from build123d import *

# Parameters (mm, degrees)
SKETCH1_R           = 50
SKETCH1_R_2         = 2.5
BOSS_EXTRUDE1_DEPTH = 3
SKETCH2_R           = 2
CUT_EXTRUDE1_DEPTH  = 4


with BuildPart() as part:
    # Sketch1 → Boss-Extrude1 (new body)
    with BuildSketch(Plane.XY):
        Circle(SKETCH1_R)
        Circle(SKETCH1_R_2, mode=Mode.SUBTRACT)
        with BuildLine():
            ThreePointArc((42, 0), (0, 42), (-42, 0))
            ThreePointArc((-42, 0), (-40, -2), (-38, 0))
            ThreePointArc((-38, 0), (0, 38), (38, 0))
            ThreePointArc((38, 0), (40, -2), (42, 0))
        make_face(mode=Mode.SUBTRACT)
    extrude(amount=BOSS_EXTRUDE1_DEPTH)

    # Sketch2 → Cut-Extrude1 (cut, through all)
    with BuildSketch(Plane.XY.offset(3)):
        with Locations((-15, 15)):
            Circle(SKETCH2_R)
        with Locations((15, 15)):
            Circle(SKETCH2_R)
        with Locations((15, -15)):
            Circle(SKETCH2_R)
        with Locations((-15, -15)):
            Circle(SKETCH2_R)
    extrude(amount=-CUT_EXTRUDE1_DEPTH, mode=Mode.SUBTRACT)


solid = part.part
Model file for the job. Use its own axes, mm. A direction names the side the tool comes from. Coordinates: 2 decimals unless noted, no trailing zeros. Loops run counter-clockwise (first coordinate to the right, second up) from the corner with the lowest first, then second, coordinate; pieces in that order, holes last. Notation, with made-up numbers: (35, 45.25) -> (93, 45.25) arc R23 cw to (93, 64.25) -> close; hole circle Ø7 at (32, 83). An arc over 180 degrees is marked (long way). Use one line per item in the form item = value. Start each with the question number.
(1) Flat gauge pins, fed straight in: pin 1 (6 mm diameter, centred on x = -25, y = 5, fed in from -Z); pin 2 (1 mm diameter, centred on y = -38.5, z = 2.5, fed in from +X). Where does each tip first touch, or does it go through?
(2) Probe probe 1 along Y at (x, z) = (15, 2.15); probe 2 along Y at (x, z) = (-4.5, 2.45); probe 3 along Y at (x, z) = (-22.5, 0.8). List the from-to ranges inside material, lowest first. Write a range as from..to.
(3) Cut at C-C on y = 6. Give the cut face in (x, z), and give its area (3 significant figures).
(4) Tool access for faces 5 (the cylindrical face through (40, -2, 1)), 6 (the flat face through (-1, -10, 0)): list every direction of +Z, -Z, +X, -X, +Y, -Y with a clear straight run to the whole face (end or side of a thin tool).
(5) Cut at B-B on z = 0.45. Give the cut face in (x, y), and give its area (3 significant figures).
(6) Pull direction Y, two halves, no side cores. Call faces 1 (the cylindrical face through (47.69, 15.02, 1.48)), 2 (the cylindrical face through (-0.54, -2.44, 1.48)), 3 (the flat face through (-1, -10, 3)), 4 (the cylindrical face through (-0.84, 37.99, 1.48)): pulls with the +Y half, pulls with the -Y half, needs draft (parallel to the pull), parting line crosses it, or undercut.
(7) Cut at A-A on x = 0. Give the cut face in (y, z), and give its area (3 significant figures).
(8) Cut at D-D on x = -40. Give the cut face in (y, z).
Values:
q1.pin_1 = 0
q1.pin_2 = 32.5
q2.probe_1 = -47.7..-17, -13..13, 17..34.91, 39.23..47.7
q2.probe_2 = -49.8..37.73, 41.76..49.8
q2.probe_3 = -44.65..30.62, 35.46..44.65
q3.outline = (-49.64, 0) -> (-41.57, 0) -> (-41.57, 3) -> (-49.64, 3) -> close; (-37.52, 0) -> (37.52, 0) -> (37.52, 3) -> (-37.52, 3) -> close; (41.57, 0) -> (49.64, 0) -> (49.64, 3) -> (41.57, 3) -> close
q3.area = 274 mm2
q4.face_5 = +Z, -Z
q4.face_6 = -Z, +X, -X, +Y, -Y
q5.outline = circle Ø100 at (0, 0); hole (-42, 0) arc R2 ccw to (-38, 0) arc R38 cw to (38, 0) arc R2 ccw to (42, 0) arc R42 ccw to start; hole circle Ø4 at (-15, -15); hole circle Ø4 at (-15, 15); hole circle Ø5 at (0, 0); hole circle Ø4 at (15, -15); hole circle Ø4 at (15, 15)
q5.area = 7,270 mm2
q6.face_1 = parting line crosses it
q6.face_2 = undercut
q6.face_3 = needs draft
q6.face_4 = undercut
q7.outline = (-50, 0) -> (-2.5, 0) -> (-2.5, 3) -> (-50, 3) -> close; (2.5, 0) -> (38, 0) -> (38, 3) -> (2.5, 3) -> close; (42, 0) -> (50, 0) -> (50, 3) -> (42, 3) -> close
q7.area = 273 mm2
q8.outline = (-30, 0) -> (-2, 0) -> (-2, 3) -> (-30, 3) -> close; (12.81, 0) -> (30, 0) -> (30, 3) -> (12.81, 3) -> close
